from build123d import *

# Parameters (mm, degrees)
F1_DEPTH = 15
F3_DEPTH = 85


with BuildPart() as f1:
    # F0 (on Top) → F1 (new body)
    with BuildSketch(Plane.XY):
        Polygon((-1097.5, 100), (1097.5, 100), (997.5, 200), (-997.5, 200), align=None)
    extrude(amount=F1_DEPTH)

    # F2 (on face) → F3 (join)
    with BuildSketch(Plane.XY.offset(15)):
        Polygon((-1097.5, 100), (1097.5, 100), (1082.5, 115), (-1082.5, 115), align=None)
    extrude(amount=F3_DEPTH)


with BuildPart() as f5_1:
    # F5: instance of F1
    add(f1.part.mirror(Plane(origin=(0, 2090.5, 50), x_dir=(1, 0, 0), z_dir=(0, -1, 0))))


solid = f5_1.part
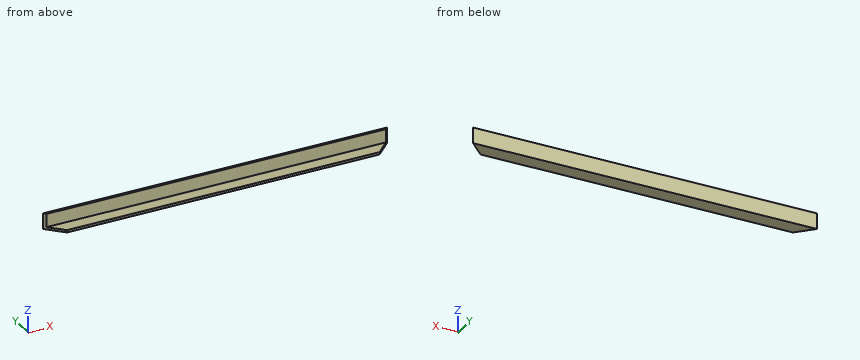
Model file for the job. Use its own axes, mm. Coordinates: 2 decimals unless noted, no trailing zeros. Loops run counter-clockwise (first coordinate to the right, second up) from the corner with the lowest first, then second, coordinate; pieces in that order, holes last. Notation, with made-up numbers: (70, -25.75) -> (84, -25.75) arc R12 ccw to (84, -11.75) -> close; hole circle Ø11 at (22, 60.5). An arc over 180 degrees is marked (long way). Use one line per item in the form item = value. Start each with the question number.
(1) Cut at B-B on x = -940. Give the cut face in (y, z).
(2) Cut at C-C on z = 58.5. Give the cut face in (x, y).
(3) Flat gauge pins, fed straight in: pin 1 (8 mm diameter, centred on y = 4062.5, z = 11, fed in from -X); pin 2 (1 mm diameter, centred on y = 4070, z = 42.5, fed in from -X). Where does each tip first touch, or does it go through?
(4) Probe probe 1 along Y at (x, z) = (-376, 23.5); probe 2 along Z at (x, y) = (-942.5, 3997.5). List the from-to ranges inside material, lowest first. Write a range as from..to.
(5) Cut at A-A on y = 4037. Give the cut face in (x, z).
Values:
q1.outline = (3981, 0) -> (4081, 0) -> (4081, 100) -> (4066, 100) -> (4066, 15) -> (3981, 15) -> close
q2.outline = (-1097.5, 4081) -> (-1082.5, 4066) -> (1082.5, 4066) -> (1097.5, 4081) -> close
q3.pin_1 = -1083
q3.pin_2 = -1087
q4.probe_1 = 4066..4081
q4.probe_2 = 0..15
q5.outline = (-1053.5, 0) -> (1053.5, 0) -> (1053.5, 15) -> (-1053.5, 15) -> close
